```python
from build123d import *

# Parameters (mm, degrees)
F0_W     = 24.8743314296
F0_H     = 5.394872278
F1_DEPTH = 5.08


with BuildPart() as f1:
    # F0 (on Top) → F1 (new body)
    with BuildSketch(Plane.XY):
        with Locations((-12.4371657148, 25.8406065404)):
            Rectangle(F0_W, F0_H)
        with Locations((12.4371657148, 25.8406065404)):
            Rectangle(F0_W, F0_H)
        Polygon((-24.8743314296, 23.1431704015), (-24.8743314296, 28.5380426794), (-29.3171685189, 28.5380426794), (-33.7600037456, 26.6339704394), (-41.0589501262, 20.9217518568), (-46.6124974191, 13.4641341865), (-43.7563844025, 13.4641341865), (-37.2508056462, 17.7482981235), (-29.3171685189, 22.3498065025), align=None)
        Polygon((29.3171685189, 28.5380426794), (24.8743314296, 28.5380426794), (24.8743314296, 23.1431704015), (29.3171685189, 22.3498065025), (37.2508056462, 17.7482981235), (43.7563844025, 13.4641341865), (46.6124974191, 13.4641341865), (41.0589501262, 20.9217518568), (33.7600037456, 26.6339704394), align=None)
    extrude(amount=F1_DEPTH)


solid = f1.part
```
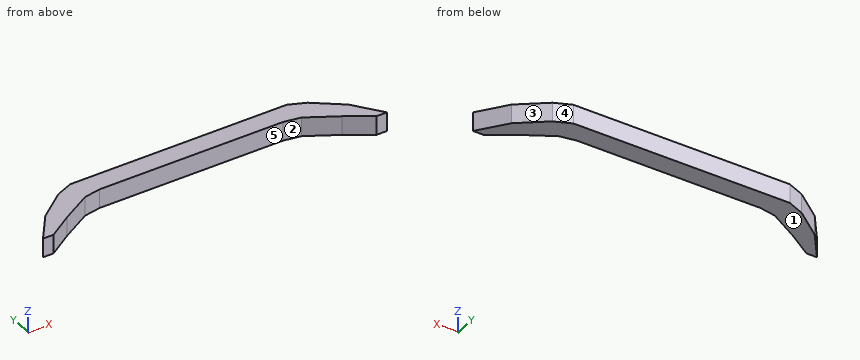
Can you work these out from the model? Positions are in its coordinate system, mm. Face numbers are marked on the shaded views. A direction names the side the tool comes from. Give positions to 0.01 mm unless a question says otherwise; leave off trailing zeros. Write each loop counter-clockwise with the first axis right and the second up, starting at its lowest first coordinate (ties: lowest second). Pieces come first, ordered by that corner, then holes. Notation, with made-up numbers: (-2.75, -7) -> (15.25, -7) arc R21 cw to (15.25, 4) -> close; hole circle Ø2 at (22.5, 81.25). An arc over 180 degrees is marked (long way). One line per item, written item: value.
Q1. For P1, Ø2.5, axis at x = 9, z = 2.5, coming from the -Y side; P2, Ø1.5, axis at y = 24.5, z = 2, coming from the -X side; P3, Ø1.5, axis at y = 20, z = 3.5, coming from the +X side, each with a flat end and sliding along its axis, tell me the tip position at first contact or that it passes through.
Results found:
P1: stops at y = 23.14
P2: stops at x = -37.45
P3: stops at x = 42.3
Q2. Imagine slicing it at B-B on z = 2. Please give me the cut outline in (x, y).
Results found:
outline: (-46.61, 13.46) -> (-43.76, 13.46) -> (-37.25, 17.75) -> (-29.32, 22.35) -> (-24.87, 23.14) -> (24.87, 23.14) -> (29.32, 22.35) -> (37.25, 17.75) -> (43.76, 13.46) -> (46.61, 13.46) -> (41.06, 20.92) -> (33.76, 26.63) -> (29.32, 28.54) -> (-29.32, 28.54) -> (-33.76, 26.63) -> (-41.06, 20.92) -> close
Q3. Imagine slicing it at D-D on y = 25. Please give me the cut outline in (x, z), and give its area (3 significant figures).
Results found:
outline: (-35.85, 0) -> (35.85, 0) -> (35.85, 5.08) -> (-35.85, 5.08) -> close
area: 364 mm^2
Q4. Imagine slicing it at C-C on x = -12.5. Please give me the cut outline in (y, z), and give its area (3 significant figures).
Results found:
outline: (23.14, 0) -> (28.54, 0) -> (28.54, 5.08) -> (23.14, 5.08) -> close
area: 27.4 mm^2
Q5. We'd pull the mould along X, two halves only. Please class the marked faces 1, 2 and 3: +X half, -X half, draft (parallel to the pull), parting line (faces both ways), or undercut.
Results found:
face 1: draft
face 2: undercut
face 3: +X half
Q6. Which directions (+Z, -Z, +X, -X, +Y, -Y) give clear straight access to the entire face, cutting with the end or side of a thin tool? Please do the marked faces 4 and 5.
Results found:
face 4: +Z, -Z, +X, +Y
face 5: +Z, -Z, -Y
Q7. Please list where these lines run through material, in increasing order: line 1 (Y direction, x = 7.5, z = 1.65); line 2 (X direction, y = 18, z = 4.25); line 3 (X direction, y = 15, z = 4.3). Write a range as [from, to].
Results found:
line 1: y = [23.14, 28.54]
line 2: x = [-43.23, -36.82], [36.82, 43.23]
line 3: x = [-45.47, -41.42], [41.42, 45.47]
Q8. Imagine slicing it at A-A on y = 19.25. Please give me the cut outline in (x, z).
Results found:
outline: (-42.3, 0) -> (-34.66, 0) -> (-34.66, 5.08) -> (-42.3, 5.08) -> close; (34.66, 0) -> (42.3, 0) -> (42.3, 5.08) -> (34.66, 5.08) -> close
